Design review of the part built by this model. Coordinates are the model's own, in mm. A direction names the side the tool comes from. Coordinates: 2 decimals unless noted, no trailing zeros. Write each loop counter-clockwise with the first axis right and the second up, starting at its lowest first coordinate (ties: lowest second). Pieces come first, ordered by that corner, then holes. Notation, with made-up numbers: M -13.75,-14.5 L 41.25,-14.5 A18 cw 41.25,-4.5 Z; hole C -33,34.5 d11. An arc over 180 degrees is marked long. Write item = value, one per line.
Autodesk Inventor part; units mm, degrees
ref_plane "YZ Plane" through (0, 0, 0) normal (1, 0, 0) x (0, 1, 0)
ref_plane "XZ Plane" through (0, 0, 0) normal (0, 1, 0) x (-1, 0, 0)
ref_plane "XY Plane" through (0, 0, 0) normal (0, 0, 1) x (1, 0, 0)
sketch "Эскиз1" plane through (0, 0, 0) normal (0, 1, 0) x (-1, 0, 0)
  circle A0 centre (0, 0) radius 15
  dimension "d0" = 30
extrude "Выдавливание1" add sketch "Эскиз1" along normal blind 55
hole "Отверстие1" at (0, 55, 0) direction (0, -1, 0) diameter 20 depth 25
hole "Отверстие2" at (0, 0, 0) direction (0, 1, 0) diameter 12 depth 30
thread "Резьба1"
chamfer "Фаска1" distance 2 angle 45 1 edges at (0, 30, -10)
chamfer "Фаска2" distance 1 angle 45 1 edges at (0, 55, -10)
equation "\"Радиус_гибки\" = Толщина"
equation "\"Ширина_просечки\" = Толщина"
equation "\"Глубина_просечки\" = 0.5 * Толщина"
equation "\"Размер_просечки\" = 4 * Толщина"
equation "\"Мин_остаток\" = 2 * Толщина"
equation "\"Радиус_перехода\" = Радиус_гибки"
equation "\"Радиус_Якоби\" = Толщина"
equation "\"Размер_зазора\" = Толщина"
properties part number "778" material "Сталь, углеродистая"
Q1. Consider section A-A, the plane z = 0. State the section outline as (x, y) points.
Check result:
outline = M -15,0 L -6,0 L -6,30 L -8,30 L -10,32 L -10,54 L -11,55 L -15,55 Z; M 6,0 L 15,0 L 15,55 L 11,55 L 10,54 L 10,32 L 8,30 L 6,30 Z
Q2. Consider section C-C, the plane y = 42. State the section outline as (x, z) points, and give its area (3 significant figures).
Check result:
outline = C 0,0 d30; hole C 0,0 d20
area = 393 mm²
Q3. For P1, Ø2, axis at y = 5.5, z = 8.5, coming from the +X side; P2, Ø6, axis at x = 5, y = 38.5, coming from the -Z side; P3, Ø1.5, axis at x = 12, y = 13, coming from the -Z side, all flat-tipped, find the tip position at first contact; note any pin that passes through.
Check result:
P1 = 12.99
P2 = -14.87
P3 = -9.92
Q4. Consider section B-B, the plane x = 0. State the section outline as (y, z) points.
Check result:
outline = M 0,-15 L 55,-15 L 55,-11 L 54,-10 L 32,-10 L 30,-8 L 30,-6 L 0,-6 Z; M 0,6 L 30,6 L 30,8 L 32,10 L 54,10 L 55,11 L 55,15 L 0,15 Z
Q5. Machinability: for faces 1 (the flat face through (0.2, 0, -6.5)), 2 (the cylindrical face through (9.76, 42.85, -2.17)), which of the approach directions +Z, -Z, +X, -X, +Y, -Y give a long, thin tool a straight path to every point of the face, cutting with its end or side? Answer none if there is none.
Check result:
face_1 = +Z, -Z, +X, -X, -Y
face_2 = +Y
Q6. Wall thickness on line 1 (Z direction, x = 0, y = 13.5); line 2 (Z direction, x = 0, y = 43.5); line 3 (Y direction, x = -1.75, z = 7): over which ranges is each line inside the solid? List them lowest first.
Check result:
line_1 = -15 to -6, 6 to 15
line_2 = -15 to -10, 10 to 15
line_3 = 0 to 30
Q7. Consider section D-D, the plane x = 12.25. State the section outline as (y, z) points.
Check result:
outline = M 0,-8.66 L 55,-8.66 L 55,8.66 L 0,8.66 Z
Q8. The part is to be moulded in two halves that separate along Z. For faces 3 (the conical face through (8.06, 30.13, -1.06)), 4 (the cylindrical face through (14.985, 27.115, -0.66)), 5 (the flat face through (5, 55, 10)), say which applies: +Z half, -Z half, draft (parallel to the pull), parting line (faces both ways), or undercut.
Check result:
face_3 = undercut
face_4 = parting line
face_5 = draft
